```python
from build123d import *

# Parameters (mm, degrees)
SKETCH1_W                = 30
SKETCH1_H                = 9
BOSS_EXTRUDE1_DEPTH      = 3
BOSS_EXTRUDE2_DEPTH      = 4
BOSS_EXTRUDE2_DEPTH_BACK = 4
SKETCH3_W                = 11
SKETCH3_H                = 2
CUT_EXTRUDE1_DEPTH       = 3
SKETCH5_R                = 1.75
CUT_EXTRUDE2_DEPTH       = 14
SKETCH6_R                = 3
CUT_EXTRUDE3_DEPTH       = 2
FILLET1_R                = 10
FILLET2_R                = 10
CHAMFER1_SIZE            = 1
FILLET3_R                = 4.5


with BuildPart() as part:
    # Sketch1 → Boss-Extrude1 (new body)
    with BuildSketch(Plane(origin=(0, 0, 0), x_dir=(1, 0, 0), z_dir=(0, 1, 0))):
        Rectangle(SKETCH1_W, SKETCH1_H)
    extrude(amount=BOSS_EXTRUDE1_DEPTH)

    # Sketch2 → Boss-Extrude2 (add, two sides: drawn at the far end of the back side and taken through both)
    with BuildSketch(Plane.XY.offset(-BOSS_EXTRUDE2_DEPTH_BACK)):
        Polygon((-15, 3), (-4, 6), (4, 6), (15, 3), align=None)
    extrude(amount=BOSS_EXTRUDE2_DEPTH + BOSS_EXTRUDE2_DEPTH_BACK)

    # Sketch3 → Cut-Extrude1 (cut)
    with BuildSketch(Plane(origin=(0, 6, 0), x_dir=(1, 0, 0), z_dir=(0, 1, 0))):
        with Locations((9.5, 3)):
            Rectangle(SKETCH3_W, SKETCH3_H)
        with Locations((-9.5, 3)):
            Rectangle(SKETCH3_W, SKETCH3_H)
        with Locations((-9.5, -3)):
            Rectangle(SKETCH3_W, SKETCH3_H)
        with Locations((9.5, -3)):
            Rectangle(SKETCH3_W, SKETCH3_H)
    extrude(amount=-CUT_EXTRUDE1_DEPTH, mode=Mode.SUBTRACT)

    # Sketch5 → Cut-Extrude2 (cut)
    with BuildSketch(Plane(origin=(0, 6, 0), x_dir=(1, 0, 0), z_dir=(0, 1, 0))):
        with Locations(Location((0, 0, 0), (0, 0, 270))):
            Circle(SKETCH5_R)
    extrude(amount=-CUT_EXTRUDE2_DEPTH, mode=Mode.SUBTRACT)

    # Sketch6 → Cut-Extrude3 (cut)
    with BuildSketch(Plane(origin=(0, 6, 0), x_dir=(1, 0, 0), z_dir=(0, 1, 0))):
        with Locations(Location((0, 0, 0), (0, 0, 270))):
            Circle(SKETCH6_R)
    extrude(amount=-CUT_EXTRUDE3_DEPTH, mode=Mode.SUBTRACT)

    # Fillet1
    # the kernel refuses this fillet: 10 mm, written as the material it adds along each edge
    with BuildSketch(Plane(origin=(-4, 21, -2), x_dir=(-1, 0, 0), z_dir=(0, -1, 0))) as fillet1_piece_1_section:
        with BuildLine():
            CenterArc((6, 10), FILLET1_R, 233.130102354, 36.869897646)
            Line((0, 2), (0, 0))
            Line((0, 0), (6, 0))
        make_face()
    fillet1_piece_1 = extrude(amount=18, mode=Mode.PRIVATE)
    fillet1_piece_1 = split(fillet1_piece_1, bisect_by=Plane(origin=(-0.192307692, 7.038461538, -2), z_dir=(0.2631174057921088, -0.9647638212377322, 0)), keep=Keep.TOP, mode=Mode.PRIVATE)
    add(fillet1_piece_1)
    with BuildSketch(Plane(origin=(4, 21, -2), x_dir=(0, 0, -1), z_dir=(0, -1, 0))) as fillet1_piece_2_section:
        with BuildLine():
            CenterArc((10, 6), FILLET1_R, 180, 36.869897646)
            Line((0, 6), (0, 0))
            Line((0, 0), (2, 0))
        make_face()
    fillet1_piece_2 = extrude(amount=18, mode=Mode.PRIVATE)
    fillet1_piece_2 = split(fillet1_piece_2, bisect_by=Plane(origin=(0.192307692, 7.038461538, -2), z_dir=(-0.2631174057921089, -0.9647638212377321, 0)), keep=Keep.TOP, mode=Mode.PRIVATE)
    add(fillet1_piece_2)
    with BuildSketch(Plane(origin=(4, 21, 2), x_dir=(1, 0, 0), z_dir=(0, -1, 0))) as fillet1_piece_3_section:
        with BuildLine():
            CenterArc((6, 10), FILLET1_R, 233.130102354, 36.869897646)
            Line((0, 2), (0, 0))
            Line((0, 0), (6, 0))
        make_face()
    fillet1_piece_3 = extrude(amount=18, mode=Mode.PRIVATE)
    fillet1_piece_3 = split(fillet1_piece_3, bisect_by=Plane(origin=(0.192307692, 7.038461538, 2), z_dir=(-0.2631174057921089, -0.9647638212377321, 0)), keep=Keep.TOP, mode=Mode.PRIVATE)
    add(fillet1_piece_3)
    with BuildSketch(Plane(origin=(-4, 21, 2), x_dir=(0, 0, 1), z_dir=(0, -1, 0))) as fillet1_piece_4_section:
        with BuildLine():
            CenterArc((10, 6), FILLET1_R, 180, 36.869897646)
            Line((0, 6), (0, 0))
            Line((0, 0), (2, 0))
        make_face()
    fillet1_piece_4 = extrude(amount=18, mode=Mode.PRIVATE)
    fillet1_piece_4 = split(fillet1_piece_4, bisect_by=Plane(origin=(-0.192307692, 7.038461538, 2), z_dir=(0.2631174057921088, -0.9647638212377322, 0)), keep=Keep.TOP, mode=Mode.PRIVATE)
    add(fillet1_piece_4)

    # Fillet2
    fillet2_edges = [part.edges().sort_by_distance(p)[0] for p in [
        (-4, 4.5, -4),
        (4, 4.5, -4),
        (4, 4.5, 4),
        (-4, 4.5, 4),
    ]]
    fillet(fillet2_edges, radius=FILLET2_R)

    # Chamfer1
    # the kernel refuses this chamfer: 1 mm, written as the material it adds along each edge
    with BuildSketch(Plane(origin=(1.282202113, 3, -4), x_dir=(0, 1, 0), z_dir=(-1, 0, 0))) as chamfer1_piece_1_section:
        Polygon((CHAMFER1_SIZE, 0), (0, CHAMFER1_SIZE), (0, 0), align=None)
    chamfer1_piece_1 = extrude(amount=2.564404226, mode=Mode.PRIVATE)
    chamfer1_piece_1 = split(chamfer1_piece_1, bisect_by=Plane(origin=(1.282202113, 3, -4.5), z_dir=(0, 0, 1)), keep=Keep.TOP, mode=Mode.PRIVATE)
    add(chamfer1_piece_1)
    with BuildSketch(Plane(origin=(10, 3, -12), x_dir=(0, 0, 1), z_dir=(1, 0, 0))) as chamfer1_piece_2:
        Polygon((10 - CHAMFER1_SIZE, 0), (10, -CHAMFER1_SIZE), (10, 0), align=None)
    revolve(axis=Axis((10, 3, -12), (0, -1, 0)), revolution_arc=25.841932763)
    with BuildSketch(Plane(origin=(1.282202113, 3, 4), x_dir=(0, 0, 1), z_dir=(-1, 0, 0))) as chamfer1_piece_3_section:
        Polygon((CHAMFER1_SIZE, 0), (0, CHAMFER1_SIZE), (0, 0), align=None)
    chamfer1_piece_3 = extrude(amount=2.564404226, mode=Mode.PRIVATE)
    chamfer1_piece_3 = split(chamfer1_piece_3, bisect_by=Plane(origin=(1.282202113, 3, 4.5), z_dir=(0, 0, -1)), keep=Keep.TOP, mode=Mode.PRIVATE)
    add(chamfer1_piece_3)
    with BuildSketch(Plane(origin=(-10, 3, 12), x_dir=(0, 0, -1), z_dir=(-1, 0, 0))) as chamfer1_piece_4:
        Polygon((10, -CHAMFER1_SIZE), (10 - CHAMFER1_SIZE, 0), (10, 0), align=None)
    revolve(axis=Axis((-10, 3, 12), (0, -1, 0)), revolution_arc=25.841932763)
    with BuildSketch(Plane(origin=(-1.282202113, 3, 6), x_dir=(0, 0, -1), z_dir=(1, 0, 0))) as chamfer1_piece_5_section:
        Polygon((10, CHAMFER1_SIZE), (10 + CHAMFER1_SIZE, 0), (10, 0), align=None)
    chamfer1_piece_5 = revolve(axis=Axis((-1.282202113, 3, 6), (0, 1, 0)), revolution_arc=25.841932763, mode=Mode.PRIVATE)
    chamfer1_piece_5 = split(chamfer1_piece_5, bisect_by=Plane(origin=(-1.282202113, 3, -4.5), z_dir=(0, 0, 1)), keep=Keep.TOP, mode=Mode.PRIVATE)
    add(chamfer1_piece_5)
    with BuildSketch(Plane(origin=(1.282202113, 3, 6), x_dir=(0, 0, -1), z_dir=(-1, 0, 0))) as chamfer1_piece_6_section:
        Polygon((10, -CHAMFER1_SIZE), (10 + CHAMFER1_SIZE, 0), (10, 0), align=None)
    chamfer1_piece_6 = revolve(axis=Axis((1.282202113, 3, 6), (0, -1, 0)), revolution_arc=25.841932763, mode=Mode.PRIVATE)
    chamfer1_piece_6 = split(chamfer1_piece_6, bisect_by=Plane(origin=(1.282202113, 3, -4.5), z_dir=(0, 0, 1)), keep=Keep.TOP, mode=Mode.PRIVATE)
    add(chamfer1_piece_6)
    with BuildSketch(Plane(origin=(1.282202113, 3, -6), x_dir=(0.43588989435406694, 0, 0.9000000000000001), z_dir=(0.9000000000000001, 0, -0.43588989435406694))) as chamfer1_piece_7_section:
        Polygon((10 + CHAMFER1_SIZE, 0), (10, -CHAMFER1_SIZE), (10, 0), align=None)
    chamfer1_piece_7 = revolve(axis=Axis((1.282202113, 3, -6), (0, -1, 0)), revolution_arc=25.841932763, mode=Mode.PRIVATE)
    chamfer1_piece_7 = split(chamfer1_piece_7, bisect_by=Plane(origin=(1.282202113, 3, 4.5), z_dir=(0, 0, -1)), keep=Keep.TOP, mode=Mode.PRIVATE)
    add(chamfer1_piece_7)
    with BuildSketch(Plane(origin=(-1.282202113, 3, -6), x_dir=(-0.4358898943539643, 0, 0.9000000000000499), z_dir=(-0.9000000000000499, 0, -0.4358898943539643))) as chamfer1_piece_8_section:
        Polygon((10, CHAMFER1_SIZE), (10 + CHAMFER1_SIZE, 0), (10, 0), align=None)
    chamfer1_piece_8 = revolve(axis=Axis((-1.282202113, 3, -6), (0, 1, 0)), revolution_arc=25.841932763, mode=Mode.PRIVATE)
    chamfer1_piece_8 = split(chamfer1_piece_8, bisect_by=Plane(origin=(-1.282202113, 3, 4.5), z_dir=(0, 0, -1)), keep=Keep.TOP, mode=Mode.PRIVATE)
    add(chamfer1_piece_8)
    with BuildSketch(Plane(origin=(-10, 3, 2), x_dir=(0, 1, 0), z_dir=(-1, 0, 0))) as chamfer1_piece_9_section:
        Polygon((CHAMFER1_SIZE, 0), (0, -CHAMFER1_SIZE), (0, 0), align=None)
    chamfer1_piece_9 = extrude(amount=5, mode=Mode.PRIVATE)
    chamfer1_piece_9 = split(chamfer1_piece_9, bisect_by=Plane(origin=(-10.346153846, 4.269230769, 2), z_dir=(0.2631174057919396, -0.9647638212377784, 0)), keep=Keep.TOP, mode=Mode.PRIVATE)
    add(chamfer1_piece_9)
    with BuildSketch(Plane(origin=(10, 3, -2), x_dir=(0, 0, -1), z_dir=(1, 0, 0))) as chamfer1_piece_10_section:
        Polygon((CHAMFER1_SIZE, 0), (0, CHAMFER1_SIZE), (0, 0), align=None)
    chamfer1_piece_10 = extrude(amount=5, mode=Mode.PRIVATE)
    chamfer1_piece_10 = split(chamfer1_piece_10, bisect_by=Plane(origin=(10.346153846, 4.269230769, -2), z_dir=(-0.2631174057919396, -0.9647638212377784, 0)), keep=Keep.TOP, mode=Mode.PRIVATE)
    add(chamfer1_piece_10)
    with BuildSketch(Plane(origin=(-15, 3, -2), x_dir=(0, 1, 0), z_dir=(1, 0, 0))) as chamfer1_piece_11_section:
        Polygon((CHAMFER1_SIZE, 0), (0, -CHAMFER1_SIZE), (0, 0), align=None)
    chamfer1_piece_11 = extrude(amount=5, mode=Mode.PRIVATE)
    chamfer1_piece_11 = split(chamfer1_piece_11, bisect_by=Plane(origin=(-15, 3, -2), z_dir=(0.2631174057919396, -0.9647638212377784, 0)), keep=Keep.TOP, mode=Mode.PRIVATE)
    add(chamfer1_piece_11)
    with BuildSketch(Plane(origin=(-10, 3, -12), x_dir=(0.43588989435406783, 0, 0.8999999999999998), z_dir=(0.8999999999999998, 0, -0.43588989435406783))) as chamfer1_piece_12:
        Polygon((10, -CHAMFER1_SIZE), (10 - CHAMFER1_SIZE, 0), (10, 0), align=None)
    revolve(axis=Axis((-10, 3, -12), (0, -1, 0)), revolution_arc=25.841932763)
    with BuildSketch(Plane(origin=(15, 3, 2), x_dir=(0, 0, 1), z_dir=(-1, 0, 0))) as chamfer1_piece_13_section:
        Polygon((CHAMFER1_SIZE, 0), (0, CHAMFER1_SIZE), (0, 0), align=None)
    chamfer1_piece_13 = extrude(amount=5, mode=Mode.PRIVATE)
    chamfer1_piece_13 = split(chamfer1_piece_13, bisect_by=Plane(origin=(15, 3, 2), z_dir=(-0.2631174057919396, -0.9647638212377784, 0)), keep=Keep.TOP, mode=Mode.PRIVATE)
    add(chamfer1_piece_13)
    with BuildSketch(Plane(origin=(10, 3, 12), x_dir=(-0.43588989435406783, 0, -0.8999999999999998), z_dir=(-0.8999999999999998, 0, 0.43588989435406783))) as chamfer1_piece_14:
        Polygon((10 - CHAMFER1_SIZE, 0), (10, -CHAMFER1_SIZE), (10, 0), align=None)
    revolve(axis=Axis((10, 3, 12), (0, -1, 0)), revolution_arc=25.841932763)

    # Fillet3
    # the kernel refuses this fillet: 4.5 mm, written as the material it takes off along each edge
    with BuildSketch(Plane(origin=(15, -11.25, -4.5), x_dir=(0, 0, 1), z_dir=(0, 1, 0)), Plane(origin=(-15, -11.25, -4.5), x_dir=(1, 0, 0), z_dir=(0, 1, 0))) as fillet3_piece_1:
        with BuildLine():
            CenterArc((FILLET3_R, -FILLET3_R), FILLET3_R, 90, 90)
            Line((0, -FILLET3_R), (0, 0))
            Line((0, 0), (FILLET3_R, 0))
        make_face()
    extrude(amount=25.5, mode=Mode.SUBTRACT)
    with BuildSketch(Plane(origin=(15, -11.25, 4.5), x_dir=(0, 0, -1), z_dir=(0, 1, 0)), Plane(origin=(-15, -11.25, 4.5), x_dir=(1, 0, 0), z_dir=(0, 1, 0))) as fillet3_piece_2:
        with BuildLine():
            CenterArc((FILLET3_R, FILLET3_R), FILLET3_R, 180, 90)
            Line((0, FILLET3_R), (0, 0))
            Line((0, 0), (FILLET3_R, 0))
        make_face()
    extrude(amount=25.5, mode=Mode.SUBTRACT)


solid = part.part
```
Could you check a few things on this model? Use its own coordinates, in mm. A direction names the side the tool comes from. Coordinates: 2 decimals unless noted, no trailing zeros. Write each loop counter-clockwise with the first axis right and the second up, starting at its lowest first coordinate (ties: lowest second). Pieces come first, ordered by that corner, then holes. Notation, with made-up numbers: M -30,71 L -2,71 A26 cw -2,110 Z; hole C 35,-31.75 d8. An arc over 180 degrees is marked long. Answer as CSV lines item,"result". Start each with the question number.
1) I want a section at B-B, the plane x = -0.75. Please give me the cut outline in (y, z).
2) I want a section at C-C, the plane y = 4.8. Please give me the cut outline in (x, z), and give its area (3 significant figures).
3) For P1, Ø4, axis at x = -9.5, z = -3, coming from the -Y side; P2, Ø2, axis at x = 0.5, y = 5.5, coming from the -Z side; P3, Ø1, axis at x = -8, z = -1, coming from the +Y side; P4, Ø1.6, axis at x = 7.5, z = -4, coming from the +Y side, each with a flat end and sliding along its axis, tell me the tip position at first contact or that it passes through.
4) For faces 4 (the flat face through (9, 3, -4)), 5 (the flat face through (-11.6, 3.4, -2.6)), 6 (the flat face through (-11.6, 3.4, 2.6)), which set-ups out of +Z, -Z, +X, -X, +Y, -Y let a thin tool reach every point of the face, with its end or its side?
5) We'd pull the mould along X, two halves only. Please class faces 1 (the flat face through (0, 5, 4)), 2 (the cylindrical face through (-15, 2, 0)), 3 (the flat face through (-2, 4, 0)): +X half, -X half, draft (parallel to the pull), parting line (faces both ways), or undercut.
6) Please list where these lines run through material, in increasing order: line 1 (X direction, y = 2.9, z = 0); line 2 (Y direction, x = -11, z = 4.25); line 3 (Z direction, x = 4, y = 4.55). Write a range as from..to.
7) I want a section at A-A, the plane y = 2.35. Please give me the cut outline in (x, z).
Data:
1,outline,"M 0,-4.5 L 3.5,-4.5 L 4,-4 L 6,-4 L 6,-2.9 L 4,-2.9 L 4,-1.58 L 0,-1.58 Z; M 0,1.58 L 4,1.58 L 4,2.9 L 6,2.9 L 6,4 L 4,4 L 3.5,4.5 L 0,4.5 Z"
2,outline,"M -8.4,-2.13 A10 cw -5.64,-3 A10 ccw -1.28,-4 L 1.28,-4 A10 ccw 5.64,-3 A10 cw 8.4,-2.13 L 8.4,2.13 A10 cw 5.64,3 A10 ccw 1.28,4 L -1.28,4 A10 ccw -5.64,3 A10 cw -8.4,2.13 Z; hole C 0,0 d6"
2,area,"83.8 mm^2"
3,P1,"stops at y = 0"
3,P2,"stops at z = -4"
3,P3,"stops at y = 5.05"
3,P4,"stops at y = 3.18"
4,face 4,"-Z, +X, +Y"
4,face 5,"-Z, -X, +Y"
4,face 6,"+Z, -X, +Y"
5,face 1,"draft"
5,face 2,"-X half"
5,face 3,"undercut"
6,line 1,"x = -15..-1.75, 1.75..15"
6,line 2,"y = 0..3"
6,line 3,"z = -3.62..3.62"
7,outline,"M -10.5,-4.5 L 10.5,-4.5 A4.5 ccw 10.5,4.5 L -10.5,4.5 A4.5 ccw Z; hole C 0,0 d3.5"
